Autodesk Inventor part; units mm, degrees
ref_plane "YZ Plane" through (0, 0, 0) normal (1, 0, 0) x (0, 1, 0)
ref_plane "XZ Plane" through (0, 0, 0) normal (0, 1, 0) x (-1, 0, 0)
ref_plane "XY Plane" through (0, 0, 0) normal (0, 0, 1) x (1, 0, 0)
sketch "Sketch1" plane through (0, 0, 0) normal (0, 1, 0) x (-1, 0, 0)
  line L0 (15, 20) -> (-15, 20)
  line L1 (-15, 20) -> (-15, -20)
  line L2 (-15, -20) -> (15, -20)
  line L3 (15, -20) -> (15, 20)
  line L4 (15, 20) -> (-15, -20) construction
  line L5 (-15, 20) -> (15, -20) construction
  point P0 (0, 0)
  dimension "d0" = 30
  dimension "d1" = 40
extrude "Extrusion1" add sketch "Sketch1" along normal blind 3
sketch "Sketch2" plane through (0, 3, 0) normal (0, 1, 0) x (1, 0, 0)
  line L0 (-15, 20) -> (-15, -20)
  line L1 (15, 20) -> (-15, 20)
  line L2 (-15, -20) -> (-3.5, -20)
  line L3 (-3.5, -20) -> (-3.5, 20)
  line L4 (-3.5, 20) -> (-15, 20)
  line L5 (-15, 20) -> (-15, -20)
  line L6 (15, -20) -> (3.5, -20)
  line L7 (3.5, -20) -> (3.5, 20)
  line L8 (3.5, 20) -> (15, 20)
  line L9 (15, 20) -> (15, -20)
  point P0 (0, 0)
  dimension "d4" = 7
  dimension "d5" = 3.5
  dimension "d6" = 15
extrude "Extrusion2" add sketch "Sketch2" along normal blind 3
sketch "Sketch3" plane through (0, 0, 0) normal (0, -1, 0) x (1, 0, 0)
  line L0 (15, -20) -> (-15, -20)
  line L1 (8.85, 20) -> (-8.85, 20)
  line L2 (-8.85, 20) -> (-8.85, -20)
  line L3 (-8.85, -20) -> (8.85, -20)
  line L4 (8.85, -20) -> (8.85, 20)
  line L5 (8.85, 20) -> (-8.85, -20) construction
  line L6 (-8.85, 20) -> (8.85, -20) construction
  point P0 (0, 0)
  dimension "d9" = 17.7
extrude "Extrusion3" add sketch "Sketch3" along normal blind 2.1
sketch "Sketch4" plane through (0, -2.1, 0) normal (0, -1, 0) x (1, 0, 0)
  line L0 (-8.85, -20) -> (-15, -20)
  line L1 (12.8, 20) -> (-12.8, 20)
  line L2 (-12.8, 20) -> (-12.8, -20)
  line L3 (-12.8, -20) -> (12.8, -20)
  line L4 (12.8, -20) -> (12.8, 20)
  line L5 (12.8, 20) -> (-12.8, -20) construction
  line L6 (-12.8, 20) -> (12.8, -20) construction
  line L7 (15, 20) -> (15, -20)
  line L8 (-12.8, -17) -> (12.8, -17)
  line L9 (8.85, -20) -> (8.85, 20)
  line L10 (8.85, -20) -> (8.85, -17)
  line L11 (-8.85, -20) -> (-8.85, -17)
  point P0 (0, 0)
  dimension "d12" = 2.2
  dimension "d15" = 3
extrude "Extrusion4" add sketch "Sketch4" along normal blind 2.2 contours L11 L8 L9 L3 | L8 L2 L1 L9 | L9 L1 L4 L8
sketch "Sketch5" plane through (0, -4.3, 0) normal (0, -1, 0) x (1, 0, 0)
  line L0 (-3.5, -20) -> (-15, -20)
  line L1 (8.85, 20) -> (-8.85, 20)
  line L2 (-8.85, 20) -> (-8.85, -20)
  line L3 (-8.85, -20) -> (8.85, -20)
  line L4 (8.85, -20) -> (8.85, 20)
  line L5 (8.85, 20) -> (-8.85, -20) construction
  line L6 (-8.85, 20) -> (8.85, -20) construction
  point P0 (0, 0)
  dimension "d16" = 17.7
extrude "Extrusion5" add sketch "Sketch5" along normal blind 2
properties part number "horok"
The listing builds one solid part. Answer for the finished solid, in the listing's coordinates (mm). A direction names the side the tool comes from. Give positions to 0.01 mm unless a question says otherwise; leave off trailing zeros. Write each loop counter-clockwise with the first axis right and the second up, starting at its lowest first coordinate (ties: lowest second). Pieces come first, ordered by that corner, then holes. Notation, with made-up numbers: M 63.5,7 L 94.5,7 A22 ccw 94.5,31 Z; hole C -11,-12.5 d1. An arc over 180 degrees is marked long. Write each question's results on one line, items separated by ' | '.
Q1. A tool of negligible diameter and unlimited length cuts with its end or side. For faces 5 (the flat face through (12, 0, 0)), 6 (the flat face through (-11, -4.3, 2)), 7 (the flat face through (-11, -2.1, 2)), from which of +Z, -Z, +X, -X, +Y, -Y can it reach the whole face along a straight path? Write none if from no direction.
Output values:
face 5: +Z, -Z, +X | face 6: +Z, -Z, -X, -Y | face 7: +Z, -Z, -X
Q2. Flat-ended cylindrical pins translate along their axes: P1, Ø3, axis at x = -11.5, z = 2, coming from the -Y side; P2, Ø5, axis at y = -3.5, z = 10, coming from the +X side; P3, Ø1.1, axis at y = -3, z = 3, coming from the -X side. Find the tip coordinate at first contact, or state that the pin passes through.
Output values:
P1: y = -4.3 | P2: x = 12.8 | P3: x = -12.8
Q3. For a pull along X with two mould halves and no side action, classify faces 1 (the flat face through (-12, 0, 0)), 2 (the flat face through (0, 3, 0)), 3 (the flat face through (-15, 3, 0)), 4 (the flat face through (-3.5, 4, 0)) as released by +X, released by -X, zero draft, split by the parting line, or undercut.
Output values:
face 1: zero draft | face 2: undercut | face 3: released by -X | face 4: undercut
Q4. Consider L1, parallel to Y at x = 10.5, z = 1.5; L2, parallel to X at y = 3.5, z = 2.5; L3, parallel to Y at x = 14, z = 15.5. Determine where each line is inside the solid, lowest interval first. Write a range as from..to.
Output values:
L1: -4.3..-2.1, 0..6 | L2: -15..-3.5, 3.5..15 | L3: 0..6
Q5. Section B-B, the plane z = -9.5 is taken. Write down the section's boundary in (x, y).
Output values:
outline: M -15,0 L -8.85,0 L -8.85,-2.1 L -12.8,-2.1 L -12.8,-4.3 L -8.85,-4.3 L -8.85,-6.3 L 8.85,-6.3 L 8.85,-4.3 L 12.8,-4.3 L 12.8,-2.1 L 8.85,-2.1 L 8.85,0 L 15,0 L 15,6 L 3.5,6 L 3.5,3 L -3.5,3 L -3.5,6 L -15,6 Z
Q6. Section D-D, the plane x = -1.5 is taken. Write down the section's boundary in (y, z), then the cut area to 3 significant figures.
Output values:
outline: M -6.3,-20 L 3,-20 L 3,20 L -6.3,20 Z | area: 372 mm2
Q7. Section A-A, the plane y = 5 is taken. Write down the section's boundary in (x, z), then the cut area to 3 significant figures.
Output values:
outline: M -15,-20 L -3.5,-20 L -3.5,20 L -15,20 Z; M 3.5,-20 L 15,-20 L 15,20 L 3.5,20 Z | area: 920 mm2
Q8. Section C-C, the plane y = -3 is taken. Write down the section's boundary in (x, z), then the cut area to 3 significant figures.
Output values:
outline: M -12.8,-17 L -8.85,-17 L -8.85,-20 L 8.85,-20 L 8.85,-17 L 12.8,-17 L 12.8,20 L -12.8,20 Z | area: 1,000 mm2
